Geometry: final body of the model. Coordinates: model frame, mm. A direction names the side the tool comes from. Give positions to 0.01 mm unless a question says otherwise; leave off trailing zeros. Write each loop counter-clockwise with the first axis right and the second up, starting at its lowest first coordinate (ties: lowest second). Pieces come first, ordered by that corner, then holes. Notation, with made-up numbers: (-16, 12.5) -> (0, 12.5) arc R18 cw to (0, 36.5) -> close; hole circle Ø7 at (-37.5, -9). An arc over 180 degrees is marked (long way). Answer as a JSON object with one key per item and string values.
from build123d import *

# Parameters (mm, degrees)
F3_DEPTH = 13.5
F5_DEPTH = 69
F7_DEPTH = 5
F8_R     = 2


with BuildPart() as f3:
    # F2 (on Top) → F3 (new body, symmetric)
    with BuildSketch(Plane.XY):
        with BuildLine():
            ThreePointArc((-12.1, -12), (-11.5142135624, -13.4142135624), (-10.1, -14))
            Line((-10.1, -14), (-9.1, -14))
            ThreePointArc((-9.1, -14), (-7.6857864376, -13.4142135624), (-7.1, -12))
            Line((-7.1, -12), (-7.1, -5))
            Line((-7.1, -5), (-5, -5))
            Line((-5, -5), (-5, -33))
            ThreePointArc((-5, -33), (-4.4142135624, -34.4142135624), (-3, -35))
            Line((-3, -35), (-2, -35))
            ThreePointArc((-2, -35), (-0.5857864376, -34.4142135624), (0, -33))
            Line((0, -33), (0, -2))
            ThreePointArc((0, -2), (-0.5857864376, -0.5857864376), (-2, 0))
            Line((-2, 0), (-7.1, 0))
            ThreePointArc((-7.1, 0), (-8.5142135624, 0.5857864376), (-9.1, 2))
            Line((-9.1, 2), (-9.1, 18))
            ThreePointArc((-9.1, 18), (-9.6857864376, 19.4142135624), (-11.1, 20))
            Line((-11.1, 20), (-12.1, 20))
            ThreePointArc((-12.1, 20), (-13.5142135624, 19.4142135624), (-14.1, 18))
            Line((-14.1, 18), (-14.1, 0.495097568))
            ThreePointArc((-14.1, 0.495097568), (-14.0756666333, 0.0024094781), (-14.0029033785, -0.4854831077))
            Line((-14.0029033785, -0.4854831077), (-12.1970966215, -9.5145168923))
            ThreePointArc((-12.1970966215, -9.5145168923), (-12.1243333667, -10.0024094781), (-12.1, -10.495097568))
            Line((-12.1, -10.495097568), (-12.1, -12))
        make_face()
    extrude(amount=F3_DEPTH, both=True)

    # F4 (on face) → F5 (join)
    with BuildSketch(Plane.YZ):
        with BuildLine():
            Line((-23.2691742077, -13.5), (-16.7308257923, -13.5))
            add(Edge.make_bspline(
                [(-16.7308257923, -13.5), (-2.7938199597, 0), (-16.7308257923, 13.5)],
                knots=[0.4510268118, 0.4510268118, 0.4510268118, 2.6905658418, 2.6905658418, 2.6905658418], degree=2, weights=[1, 0.4358898944, 1]))
            Line((-16.7308257923, 13.5), (-23.2691742077, 13.5))
            add(Edge.make_bspline(
                [(-23.2691742077, 13.5), (-37.2061800403, 0), (-23.2691742077, -13.5)],
                knots=[3.5926194654, 3.5926194654, 3.5926194654, 5.8321584954, 5.8321584954, 5.8321584954], degree=2, weights=[1, 0.4358898944, 1]))
        make_face()
        with BuildLine():
            Line((-16.7308257923, -13.5), (-13.4616515847, -13.5))
            ThreePointArc((-13.4616515847, -13.5), (-5, 0), (-13.4616515847, 13.5))
            Line((-13.4616515847, 13.5), (-16.7308257923, 13.5))
            add(Edge.make_bspline(
                [(-16.7308257923, -13.5), (-2.7938199597, 0), (-16.7308257923, 13.5)],
                knots=[0.4510268118, 0.4510268118, 0.4510268118, 2.6905658418, 2.6905658418, 2.6905658418], degree=2, weights=[1, 0.4358898944, 1]))
        make_face()
    extrude(amount=F5_DEPTH)

    # F6 (on face) → F7 (join)
    with BuildSketch(Plane.YZ.offset(69)):
        with BuildLine():
            Line((-10.4616515847, 13.5), (-13.4616515847, 13.5))
            ThreePointArc((-13.4616515847, 13.5), (-5, 0), (-13.4616515847, -13.5))
            Line((-13.4616515847, -13.5), (-10.4616515847, -13.5))
            ThreePointArc((-10.4616515847, -13.5), (-2, 0), (-10.4616515847, 13.5))
        make_face()
    extrude(amount=-F7_DEPTH)

    # F8
    f8_edges = [f3.edges().sort_by_distance(p)[0] for p in [
        (0, -5, 0),
        (0, -27.5, -0.000816),
        (64, -5, 0),
    ]]
    fillet(f8_edges, radius=F8_R)


solid = f3.part
Q1. Cut plane A-A (y = -22). Return the cut outline in (x, z).
Values:
{"outline": "(-5, -13.5) -> (69, -13.5) -> (69, 13.5) -> (-5, 13.5) -> close"}
Q2. Set-up query: faces 1 (the flat face through (-9.1, 10, 0)), 2 (the cylindrical face through (-7.7, -13.43, 0.19)), 3 (the flat face through (0, -2.7, 0.1)). Return all of +Z, -Z, +X, -X, +Y, -Y with unobstructed straight access to the full face (end or side cutting, diameter ignored); none if empty.
Values:
{"face 1": "+Z, -Z, +X, +Y", "face 2": "+Z, -Z, -Y", "face 3": "+Y"}
Q3. Material intervals for L1, parallel to Y at x = -5.5, z = 9.5; L2, parallel to X at y = 16.5, z = -8.25; L3, parallel to X at y = -19.5, z = -0.25, sorted ascending. Write a range as from..to.
Values:
{"L1": "-5..0", "L2": "-14.1..-9.1", "L3": "-5..69"}
Q4. First-contact query: P1, Ø3, axis at x = 32, y = -7.5, coming from the +Z side; P2, Ø8, axis at x = 33.5, z = 2, coming from the -Y side; P3, Ø1.1, axis at x = -9.5, z = 0, coming from the -Y side. Flat tips, straight axial feed; report the tip coordinate or a pass-through.
Values:
{"P1": "z = 10.2", "P2": "y = -27.5", "P3": "y = -14"}
Q5. Mould query, pull axis X, two halves, no side actions, for faces 4 (the flat face through (64, -2.8, 0.1)), 5 (the cylindrical face through (-13.5, 19.43, 0.19)), 6 (the cylindrical face through (-8.5, 0.57, 0.19)). Classes: pulls with the +X half, pulls with the -X half, needs draft (parallel to the pull), parting line crosses it, or undercut.
Values:
{"face 4": "undercut", "face 5": "pulls with the -X half", "face 6": "pulls with the +X half"}
Q6. Cut plane B-B (x = -1). Return the cut outline in (y, z), and give its area (3 significant figures).
Values:
{"outline": "(-34.73, -13.5) -> (-0.27, -13.5) -> (-0.27, 13.5) -> (-34.73, 13.5) -> close", "area": "931 mm²"}
